Input: part model. Units: mm. Frame: model coordinates. Face numbers are marked on the shaded views. A direction names the side the tool comes from. Give positions to 0.01 mm unless a question says otherwise; leave off trailing zeros. Order: outer loops, then holes, each group sorted by start corner. A loop starts at its lowest first (then second) coordinate and runs counter-clockwise, first axis right, second up. Notation, with made-up numbers: (-28, -12) - (10, -12) arc R20 cw to (10, 22) - close; hole circle Ø3 at (-15.5, 15.25). An arc over 180 degrees is marked (long way). Use a Markdown table: item, result.
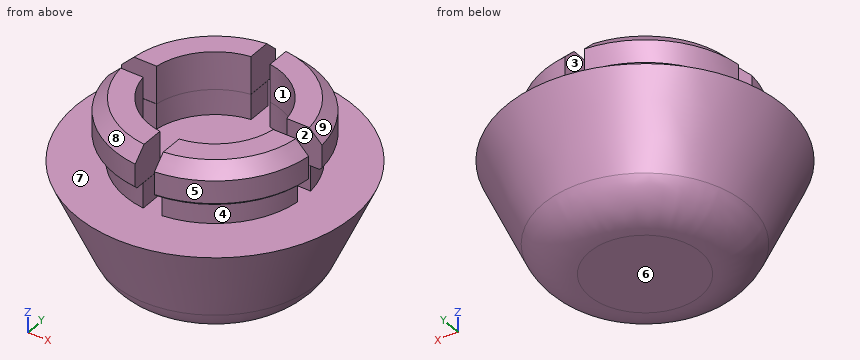
from build123d import *

# Parameters (mm, degrees)
F1_R     = 8.89
F2_R     = 13.97
F5_R     = 5.08
F7_DEPTH = 2.54
F9_DEPTH = 3.81
F10_SIZE = 1.27
F11_SIZE = 0.254


with BuildPart() as f4:
    # F1 (on Top) → F4 section 0
    with BuildSketch(Plane.XY):
        Circle(F1_R)
    # F2 (on offset) → F4 section 1
    with BuildSketch(Plane.XY.offset(11.43)):
        Circle(F2_R)
    loft()

    # F5
    f5_edges = [f4.edges().sort_by_distance(p)[0] for p in [
        (-8.89, 0, 0),
    ]]
    fillet(f5_edges, radius=F5_R)

    # F6 (on offset) → F7 (join)
    with BuildSketch(Plane.XY.offset(11.43)):
        with BuildLine():
            Line((-0.9525, 6.5696794791), (-0.9525, 8.9808006413))
            ThreePointArc((-0.9525, 8.9808006413), (-6.3860017386, 6.3860017386), (-8.9808006413, 0.9525))
            Line((-8.9808006413, 0.9525), (-6.5696794791, 0.9525))
            ThreePointArc((-6.5696794791, 0.9525), (-4.694035828, 4.694035828), (-0.9525, 6.5696794791))
        make_face()
        with BuildLine():
            ThreePointArc((-0.9525, -6.5696794791), (-4.694035828, -4.694035828), (-6.5696794791, -0.9525))
            Line((-6.5696794791, -0.9525), (-8.9808006413, -0.9525))
            ThreePointArc((-8.9808006413, -0.9525), (-6.3860017386, -6.3860017386), (-0.9525, -8.9808006413))
            Line((-0.9525, -8.9808006413), (-0.9525, -6.5696794791))
        make_face()
        with BuildLine():
            ThreePointArc((0.9525, -8.9808006413), (6.3860017386, -6.3860017386), (8.9808006413, -0.9525))
            Line((8.9808006413, -0.9525), (6.5696794791, -0.9525))
            ThreePointArc((6.5696794791, -0.9525), (4.694035828, -4.694035828), (0.9525, -6.5696794791))
            Line((0.9525, -6.5696794791), (0.9525, -8.9808006413))
        make_face()
        with BuildLine():
            Line((6.5696794791, 0.9525), (8.9808006413, 0.9525))
            ThreePointArc((8.9808006413, 0.9525), (6.3860017386, 6.3860017386), (0.9525, 8.9808006413))
            Line((0.9525, 8.9808006413), (0.9525, 6.5696794791))
            ThreePointArc((0.9525, 6.5696794791), (4.694035828, 4.694035828), (6.5696794791, 0.9525))
        make_face()
    extrude(amount=F7_DEPTH)

    # F8 (on offset) → F9 (join)
    with BuildSketch(Plane.XY.offset(13.97)):
        with BuildLine():
            Line((-0.9671329128, 6.5584753021), (-0.9671329128, 10.1138644409))
            ThreePointArc((-0.9671329128, 10.1138644409), (-7.1842048969, 7.1842048969), (-10.1138644409, 0.9671329128))
            Line((-10.1138644409, 0.9671329128), (-6.5584753021, 0.9671329128))
            ThreePointArc((-6.5584753021, 0.9671329128), (-4.6876936952, 4.6876936952), (-0.9671329128, 6.5584753021))
        make_face()
        with BuildLine():
            ThreePointArc((10.1138644409, 0.9671329128), (7.1842048969, 7.1842048969), (0.9671329128, 10.1138644409))
            Line((0.9671329128, 10.1138644409), (0.9671329128, 6.5584753021))
            ThreePointArc((0.9671329128, 6.5584753021), (4.6876936952, 4.6876936952), (6.5584753021, 0.9671329128))
            Line((6.5584753021, 0.9671329128), (10.1138644409, 0.9671329128))
        make_face()
        with BuildLine():
            ThreePointArc((0.9671329128, -10.1138644409), (7.1842048969, -7.1842048969), (10.1138644409, -0.9671329128))
            Line((10.1138644409, -0.9671329128), (6.5584753021, -0.9671329128))
            ThreePointArc((6.5584753021, -0.9671329128), (4.6876936952, -4.6876936952), (0.9671329128, -6.5584753021))
            Line((0.9671329128, -6.5584753021), (0.9671329128, -10.1138644409))
        make_face()
        with BuildLine():
            Line((-6.5584753021, -0.9671329128), (-10.1138644409, -0.9671329128))
            ThreePointArc((-10.1138644409, -0.9671329128), (-7.1842048969, -7.1842048969), (-0.9671329128, -10.1138644409))
            Line((-0.9671329128, -10.1138644409), (-0.9671329128, -6.5584753021))
            ThreePointArc((-0.9671329128, -6.5584753021), (-4.6876936952, -4.6876936952), (-6.5584753021, -0.9671329128))
        make_face()
    extrude(amount=F9_DEPTH)

    # F10
    f10_edges = [f4.edges().sort_by_distance(p)[0] for p in [
        (-7.184205, -7.184205, 17.78),
        (7.184205, -7.184205, 17.78),
        (7.184205, 7.184205, 17.78),
        (-7.184205, 7.184205, 17.78),
    ]]
    chamfer(f10_edges, length=F10_SIZE)

    # F11
    f11_edges = [f4.edges().sort_by_distance(p)[0] for p in [
        (-7.184205, -7.184205, 13.97),
        (-7.184205, 7.184205, 13.97),
        (7.184205, -7.184205, 13.97),
        (7.184205, 7.184205, 13.97),
    ]]
    chamfer(f11_edges, length=F11_SIZE)


solid = f4.part
1. Set-up query: the marked faces 1, 2, 3, 4 and 5. Return all of +Z, -Z, +X, -X, +Y, -Y with unobstructed straight access to the full face (end or side cutting, diameter ignored); none if empty.
Response:
| item | result |
|---|---|
| face 1 | +Z |
| face 2 | +Z, +X, -X |
| face 3 | +Z, +Y, -Y |
| face 4 | +X, -Y |
| face 5 | +Z, +X, -Y |
2. Section query B-B (z = 5.5). Return loops of the section in (x, y).
Response:
| item | result |
|---|---|
| outline | circle Ø22.67 at (0, 0) |
3. Pin query (flat end, axial travel): pin 1 (3 mm diameter, centred on x = 9.5, y = -10.5, fed in from -Z); pin 2 (1.5 mm diameter, centred on y = -5.5, z = 9, fed in from +X); pin 3 (0.7 mm diameter, centred on y = 8, z = 13, fed in from -X). Return the tip coordinate at first contact, or that it passes through.
Response:
| item | result |
|---|---|
| pin 1 | stops at z = 8.48 |
| pin 2 | stops at x = 12.15 |
| pin 3 | stops at x = -4.8 |
4. Mould query, pull axis Y, two halves, no side actions, for the marked faces 6, 7, 8 and 9. Classes: pulls with the +Y half, pulls with the -Y half, needs draft (parallel to the pull), parting line crosses it, or undercut.
Response:
| item | result |
|---|---|
| face 6 | needs draft |
| face 7 | undercut |
| face 8 | pulls with the -Y half |
| face 9 | pulls with the +Y half |
5. Section query C-C (z = 11). Return loops of the section in (x, y).
Response:
| item | result |
|---|---|
| outline | circle Ø27.56 at (0, 0) |
6. Material intervals for line 1 along X through (y, z) = (-1, 14.75); line 2 along Z through (x, y) = (3.75, -2); line 3 along Y through (x, z) = (2, 15.5), sorted ascending.
Response:
| item | result |
|---|---|
| line 1 | x = -10.11 to -6.55, 6.55 to 10.11 |
| line 2 | z = 0 to 11.43 |
| line 3 | y = -9.96 to -6.32, 6.32 to 9.96 |
7. Section query A-A (x = 0). Return loops of the section in (y, z), then the cut area to 3 significant figures.
Response:
| item | result |
|---|---|
| outline | (-13.97, 11.43) - (-10.23, 3.02) arc R5.08 ccw to (-5.59, 0) - (5.59, 0) arc R5.08 ccw to (10.23, 3.02) - (13.97, 11.43) - close |
| area | 257 mm^2 |
